Can you work these out from the model? Positions are in its coordinate system, mm. A direction names the side the tool comes from. Round coordinates to 2 decimals unless told otherwise and drop trailing zeros. Write each loop counter-clockwise with the first axis right and the second up, starting at its lowest first coordinate (ties: lowest second). Pieces come first, ordered by that corner, then holes. Notation, with made-up numbers: (-13, 30.5) -> (36, 30.5) arc R25 ccw to (36, 69.5) -> close; hole circle Ø4 at (65, 70.5). An arc over 180 degrees is marked (long way). Write item = value, one per line. Start each with the question number.
1) If I drill on line 1 (Y direction, x = 0, z = -3.95) (3 decimals); line 2 (X direction, y = 0, z = -0.95) (3 decimals); line 3 (Y direction, x = 4.5, z = -5), over which ranges is the centre line in solid material (lowest first)?
2) Imagine slicing it at A-A, the plane x = 0. Please give me the cut outline in (y, z) (3 decimals).
3) Thinking about a two-plate mould opening in X: for faces 4 (the face through (-0.699, 18.687, -1.121)), 5 (the face through (-4, -4, -1.75)), 6 (the face through (0, -8, -2.6)), 7 (the face through (10.353, 6.232, -1.282)), which applies, +X half, -X half, draft (parallel to the pull), parting line (faces both ways), or undercut?
4) I'm going to push flat-ended pins straight in: pin 1 (0.6 mm diameter, centred on x = 3.5, y = 3.5, fed in from +Z); pin 2 (6.5 mm diameter, centred on x = 14, y = 6, fed in from -Z); pin 3 (2 mm diameter, centred on x = -13.35, y = 6.1, fed in from +Z); pin 4 (5.5 mm diameter, centred on x = 13.35, y = 6.1, fed in from -Z). Where does each tip first touch, or does it pass through?
5) Imagine slicing it at C-C, the plane z = -4. Please give me the cut outline in (x, y) (3 decimals), then the cut area to 3 significant figures.
6) For faces 1 (the face through (0, 10, -1)), 2 (the face through (-0.054, -5.267, 0.042)), 3 (the face through (-16.347, 6.232, -1.282)), which set-ups out of +Z, -Z, +X, -X, +Y, -Y let a thin tool reach every point of the face, with its end or its side?
7) Imagine slicing it at B-B, the plane x = -13.35. Please give me the cut outline in (y, z), then the cut area to 3 significant figures.
8) Imagine slicing it at D-D, the plane y = -11.5. Please give me the cut outline in (x, z).
Autodesk Inventor part; units mm, degrees
ref_plane "YZ Plane" through (0, 0, 0) normal (1, 0, 0) x (0, 1, 0)
ref_plane "XZ Plane" through (0, 0, 0) normal (0, 1, 0) x (-1, 0, 0)
ref_plane "XY Plane" through (0, 0, 0) normal (0, 0, 1) x (1, 0, 0)
sketch "Náčrt1" plane through (0, 0, 0) normal (0, 0, 1) x (1, 0, 0)
  circle A0 centre (0, 0) radius 5.125
  arc A1 (8.5, -16.6565) -> (-8.5, -16.6565) centre (0, 0) ccw
  line L0 (-13.35, 6.1) -> (13.35, 6.1)
  line L1 (0, 18.7) -> (0, -18.7)
  line L2 (8.5, -16.6565) -> (8.5, -22.2)
  line L3 (8.5, -22.2) -> (-8.5, -22.2)
  line L4 (-8.5, -22.2) -> (-8.5, -16.6565)
  line L5 (0, -18.7) -> (8.5, -22.2) construction
  line L6 (0, -18.7) -> (-8.5, -22.2) construction
  circle A2 centre (-13.35, 6.1) radius 1.7
  circle A3 centre (13.35, 6.1) radius 1.7
  line L7 (-12.1033, 10) -> (12.1033, 10)
  arc A4 (12.1033, 10) -> (-12.1033, 10) centre (0, 0) ccw
  line L8 (4.2, 4.2) -> (-4.2, 4.2)
  line L9 (-4.2, 4.2) -> (-4.2, -4.2)
  line L10 (-4.2, -4.2) -> (4.2, -4.2)
  line L11 (4.2, -4.2) -> (4.2, 4.2)
  line L12 (4.2, 4.2) -> (-4.2, -4.2) construction
  line L13 (-4.2, 4.2) -> (4.2, -4.2) construction
  line L14 (-3.55, -20.2) -> (3.55, -20.2)
  line L15 (3.55, -20.2) -> (3.55, -17.1)
  line L16 (3.55, -17.1) -> (-3.55, -17.1)
  line L17 (-3.55, -17.1) -> (-3.55, -20.2)
  line L18 (-3.55, -20.2) -> (3.55, -17.1) construction
  line L19 (3.55, -20.2) -> (-3.55, -17.1) construction
  circle A5 centre (0, 0) radius 5.575
  circle A6 centre (0, 0) radius 18.7
  circle A7 centre (-13.35, 6.1) radius 3
  circle A8 centre (13.35, 6.1) radius 3
  point P0 (-10.088, 6.1)
  point P1 (4.2, -2.9369)
  point P2 (2.9369, -4.2)
  point P3 (-2.9369, -4.2)
  point P4 (-4.2, -2.9369)
  point P5 (-4.2, 2.9369)
  point P6 (-2.9369, 4.2)
  point P7 (4.2, 2.9369)
  point P8 (2.9369, 4.2)
  point P9 (0, -18.65)
  point P10 (-8.5, -16.6565)
  dimension "d0" = 10.25
  dimension "d1" = 37.4
  dimension "d2" = 26.7
  dimension "d3" = 17
  dimension "d5" = 22.2
  dimension "d7" = 6.1
  dimension "d9" = 3.4
  dimension "d10" = 3.4
  dimension "d12" = 10
  dimension "d14" = 3
  dimension "d25" = 8.4
  dimension "d26" = 8.4
  dimension "d31" = 3.1
  dimension "d32" = 7.1
  dimension "d33" = 2
  dimension "d39" = 0.45
  dimension "d40" = 6
  dimension "d41" = 6
extrude "Vysunutí1" add sketch "Náčrt1" along normal blind 0.4 contours A0 L11 A5 | A0 L8 A5 L11 | L11 A5 L10 A0 | A0 L1 A5 L8 | A5 L8 L11 | L11 L8 A5 L1 L7 A4 A1 A6 L15 L16 L10 | L10 A5 L1 A0 | L11 L10 A5 | A0 L8 A5 L1 | L1 A5 L10 A0 | A0 L9 A5 L8 | A5 L8 L9 L10 L1 L16 L17 A6 A1 A4 L7 | L10 A5 L9 A0 | A0 L9 A5 | A5 L9 L8 | L10 L9 A5 | L16 L15 A6 L1 | L1 A6 L17 L16 | A7 | A8
extrude "Vysunutí2" add sketch "Náčrt1" against normal blind 2.6 contours A0 L11 A5 | A0 L8 A5 L11 | L11 A5 L10 A0 | A0 L1 A5 L8 | A5 L8 L11 | L11 L8 A5 L1 L7 A4 A1 A6 L15 L16 L10 | L10 A5 L1 A0 | L11 L10 A5 | A0 L8 A5 L1 | L1 A5 L10 A0 | A0 L9 A5 L8 | A5 L8 L9 L10 L1 L16 L17 A6 A1 A4 L7 | L10 A5 L9 A0 | A0 L9 A5 | A5 L9 L8 | L10 L9 A5 | L16 L15 A6 L1 | L1 A6 L17 L16
fillet "Zaoblení1" radius 1.5 4 edges at (12.1033, 10, 0.2) (12.1033, 10, -1.3) (-12.1033, 10, 0.2) (-12.1033, 10, -1.3)
chamfer "Zkosení1" distance 0.5 angle 45 1 edges at (-5.125, 0, 0.4)
extrude "Vysunutí3" cut sketch "Náčrt1" along normal blind 0.75 and the other way blind 1.75 contours A0 L8 A5 L11 | L11 A5 L10 A0 | A5 L8 L11 | L11 L10 A5 | A0 L9 A5 L8 | L10 A5 L9 A0 | A5 L9 L8 | L10 L9 A5
sketch "Náčrt2" plane through (0, 0, -2.6) normal (0, 0, -1) x (-1, 0, 0)
  circle A0 centre (0, 0) radius 5.125
  circle A1 centre (0, 0) radius 5.7
  dimension "d35" = 11.4
extrude "Vysunutí4" add sketch "Náčrt2" along normal blind 3
fillet "Zaoblení4" radius 0.5 1 edges at (5.7, 0, -2.6)
properties part number "Držák-Cam+ir"
Reported:
q1.line_1 = -5.7 to -5.125, 5.125 to 5.7
q1.line_2 = -18.7 to -5.125, 5.125 to 18.7
q1.line_3 = -3.5 to -2.45, 2.45 to 3.5
q2.outline = (-18.7, -2.6) -> (-6.2, -2.6) arc R0.5 cw to (-5.7, -3.1) -> (-5.7, -5.6) -> (-5.125, -5.6) -> (-5.125, -0.1) -> (-5.625, 0.4) -> (-18.7, 0.4) -> close; (5.125, -5.6) -> (5.7, -5.6) -> (5.7, -3.1) arc R0.5 cw to (6.2, -2.6) -> (10, -2.6) -> (10, 0.4) -> (5.625, 0.4) -> (5.125, -0.1) -> close; (15.7, -2.6) -> (18.7, -2.6) -> (18.7, 0.4) -> (15.7, 0.4) -> close
q3.face_4 = parting line
q3.face_5 = undercut
q3.face_6 = draft
q3.face_7 = undercut
q4.pin_1 = -1.75
q4.pin_2 = -2.6
q4.pin_3 = through
q4.pin_4 = 0
q5.outline = circle Ø11.4 at (0, 0); hole circle Ø10.25 at (0, 0)
q5.area = 19.6 mm²
q6.face_1 = +Z, -Z
q6.face_2 = +Z
q6.face_3 = -Z
q7.outline = (-13.09, -2.6) -> (3.1, -2.6) -> (3.1, 0) -> (4.4, 0) -> (4.4, 0.4) -> (-13.09, 0.4) -> close; (7.8, 0) -> (9.1, 0) -> (9.1, -2.6) -> (13.09, -2.6) -> (13.09, 0.4) -> (7.8, 0.4) -> close
q7.area = 61.6 mm²
q8.outline = (-14.75, -2.6) -> (14.75, -2.6) -> (14.75, 0.4) -> (-14.75, 0.4) -> close
